Could you check a few things on this model? Use its own coordinates, in mm. A direction names the side the tool comes from. Coordinates: 2 decimals unless noted, no trailing zeros. Write each loop counter-clockwise with the first axis right and the second up, starting at its lowest first coordinate (ties: lowest second). Pieces come first, ordered by that corner, then holes.
```python
from build123d import *
from OCP.BRepFilletAPI import BRepFilletAPI_MakeChamfer

# Parameters (mm, degrees)
BOSS_EXTRUDE1_DEPTH     = 55
CUT_EXTRUDE2_DEPTH      = 206.91260281973967
CUT_EXTRUDE2_DEPTH_BACK = 206.91260281973967
SKETCH2_W               = 100.40000000000003
SKETCH2_H               = 20.399999999999995
CUT_EXTRUDE3_DEPTH      = 19
CUT_EXTRUDE4_DEPTH      = 206.91260281973967
CUT_EXTRUDE4_DEPTH_BACK = 206.91260281973967
CUT_EXTRUDE12_DEPTH     = 206.91260281973967
BOSS_EXTRUDE2_DEPTH     = 55
CHAMFER1_SIZE           = 14.54
CHAMFER1_SIZE2          = 14.538004892432124
CHAMFER8_SIZE           = 14.54
CHAMFER8_SIZE2          = 14.541995746543376
CHAMFER10_SIZE          = 3
CHAMFER10_SIZE2         = 1.732050807568882
BOSS_EXTRUDE4_DEPTH     = 55
SKETCH39_R              = 1.949999999999999
CUT_EXTRUDE13_DEPTH     = 11
SKETCH40_R              = 2.3000000000000105
SKETCH40_R_2            = 2.2999999999999985
CUT_EXTRUDE14_DEPTH     = 212.78054679313647
SKETCH41_R              = 2.2999999999999927
SKETCH41_R_2            = 2.300000000000006
CUT_EXTRUDE15_DEPTH     = 212.78054679313647
SKETCH42_R              = 5.000000000000005
SKETCH42_R_2            = 5.000000000000004
SKETCH42_R_3            = 4.99999999999999
CUT_EXTRUDE16_DEPTH     = 214.57902518739957
CHAMFER6_SIZE           = 1
CHAMFER13_SIZE          = 2
CHAMFER14_SIZE          = 4
SKETCH35_R              = 2.3
SKETCH35_R_2            = 2.3000000000000007
CUT_EXTRUDE11_DEPTH     = 157.6455394949968
CHAMFER15_SIZE          = 1
CHAMFER12_SIZE          = 2


with BuildPart() as part:
    # Sketch1 → Boss-Extrude1 (new body)
    with BuildSketch(Plane(origin=(0, 0, 0), x_dir=(1, 0, 0), z_dir=(0, 1, 0))):
        Polygon((0, 0), (149.99999999999937, 0), (74.99999999999966, 129.903810567666), align=None)
    extrude(amount=-BOSS_EXTRUDE1_DEPTH)

    # Sketch4 → Cut-Extrude2 (cut, two sides: drawn at the far end of the back side and taken through both)
    with BuildSketch(Plane(origin=(0, 0, 0), x_dir=(1, 0, 0), z_dir=(0, 1, 0)).offset(-CUT_EXTRUDE2_DEPTH_BACK)):
        Polygon((58.51197371389166, 45.56656990669255), (40.84586371751368, 35.365170120590925), (51.0472635036153, 17.699060124212945), (68.71337349999328, 27.90045991031457), align=None)
    extrude(amount=CUT_EXTRUDE2_DEPTH + CUT_EXTRUDE2_DEPTH_BACK, mode=Mode.SUBTRACT)

    # Sketch2 → Cut-Extrude3 (cut)
    with BuildSketch(Plane(origin=(0, 0, 0), x_dir=(1, 0, 0), z_dir=(0, 1, 0))):
        Polygon((109.19704525612455, 138.33483042000623), (58.99704525612457, 51.385879880048556), (41.33012701892186, 61.58587988004866), (91.53012701892203, 148.5348304200062), align=None)
        with Locations((124.20000000000002, 15.199999999999998)):
            Rectangle(SKETCH2_W, SKETCH2_H)
    extrude(amount=-CUT_EXTRUDE3_DEPTH, mode=Mode.SUBTRACT)

    # Sketch27 → Cut-Extrude4 (cut, two sides: drawn at the far end of the back side and taken through both)
    with BuildSketch(Plane(origin=(0, 0, 0), x_dir=(1, 0, 0), z_dir=(0, 1, 0)).offset(-CUT_EXTRUDE4_DEPTH_BACK)):
        Polygon((263.2126301054118, 395.09764853640723), (92.55144818336423, 99.50381056766552), (63.425446507958185, 49.05609584452599), (74.19851948196656, 30.4), (132.44855181663485, 30.400000000000006), (473.7709156607301, 30.40000000000005), (1064.9585915982134, 371.72236384409547), (854.4003060428951, 736.4200123805026), align=None)
    extrude(amount=CUT_EXTRUDE4_DEPTH + CUT_EXTRUDE4_DEPTH_BACK, mode=Mode.SUBTRACT)

    # Sketch36 → Cut-Extrude12 (cut, through all)
    with BuildSketch(Plane(origin=(0, 0, 0), x_dir=(1, 0, 0), z_dir=(0, 1, 0))):
        Polygon((0, 0), (27.744423358828314, 48.054750884192224), (55.49392370110368, 0), align=None)
    extrude(amount=-CUT_EXTRUDE12_DEPTH, mode=Mode.SUBTRACT)

    # Sketch37 → Boss-Extrude2 (add)
    with BuildSketch(Plane(origin=(0, 0, 0), x_dir=(1, 0, 0), z_dir=(0, 1, 0))):
        Polygon((34.51566032896974, 36.328770172306804), (61.707613950845634, 52.03092474503183), (75.90956267267339, 27.436928475564457), (48.717609050797485, 11.734773902839414), align=None)
        Polygon((58.51197371389166, 45.56656990669254), (40.84586371751368, 35.365170120590925), (51.0472635036153, 17.699060124212945), (68.71337349999328, 27.90045991031457), align=None, mode=Mode.SUBTRACT)
    extrude(amount=BOSS_EXTRUDE2_DEPTH)

    # Chamfer1
    chamfer1_edges = [part.edges().sort_by_distance(p)[0] for p in [
        (27.744423358828314, -27.499999999999996, -48.054750884192224),
    ]]
    chamfer1_side = [part.faces().sort_by_distance(p)[0] for p in [
        (41.61831404888806, -8.880686552520038, -24.028863834628613),
    ]]
    chamfer(chamfer1_edges, length=CHAMFER1_SIZE, length2=CHAMFER1_SIZE2, reference=chamfer1_side[0])

    # Chamfer8
    chamfer8_edges = [part.edges().sort_by_distance(p)[0] for p in [
        (55.49392370110368, -27.5, 0),
    ]]
    chamfer8_side = [part.faces().sort_by_distance(p)[0] for p in [
        (43.89644444718681, -5.451869149628209, -20.083748159692625),
    ]]
    chamfer(chamfer8_edges, length=CHAMFER8_SIZE, length2=CHAMFER8_SIZE2, reference=chamfer8_side[0])

    # Chamfer10: one chamfer whose edges measure the first distance from different faces: ONE call of the kernel's chamfer builder (chamfer() names one face for all edges)
    chamfer10_edges_1 = [part.edges().sort_by_distance(p)[0] for p in [
        (41.619173529966076, 55, -24.027375442095966),
    ]]
    chamfer10_side_1 = [part.faces().sort_by_distance(p)[0] for p in [
        (41.61917352996608, 4.8e-16, -24.02737544209596),
    ]]
    chamfer10_edges_2 = [part.edges().sort_by_distance(p)[0] for p in [
        (68.80858831175951, 55, -39.73392661029814),
    ]]
    chamfer10_side_2 = [part.faces().sort_by_distance(p)[0] for p in [
        (68.81005262159329, 3.7755355816469027, -39.731390815296024),
    ]]
    chamfer10 = BRepFilletAPI_MakeChamfer(part.part.solid().wrapped)
    for e in chamfer10_edges_1:
        chamfer10.Add(CHAMFER10_SIZE, CHAMFER10_SIZE2, e.wrapped, chamfer10_side_1[0].wrapped)  # the first distance lies on this face
    for e in chamfer10_edges_2:
        chamfer10.Add(CHAMFER10_SIZE, CHAMFER10_SIZE2, e.wrapped, chamfer10_side_2[0].wrapped)  # the first distance lies on this face
    add(Compound.cast(chamfer10.Shape()), mode=Mode.REPLACE)

    # Sketch28 → Boss-Extrude4 (add)
    with BuildSketch(Plane(origin=(0, 0, 0), x_dir=(1, 0, 0), z_dir=(0, 1, 0))):
        Polygon((63.4254465079582, 49.05609584452599), (78.17205931308985, 74.59797846255982), (85.54536553049708, 61.82937401563315), align=None)
        Polygon((103.69444359160526, 30.4), (74.19851948196656, 30.4), (96.31843850450542, 43.173278171107164), align=None)
    extrude(amount=-BOSS_EXTRUDE4_DEPTH)

    # Sketch39 → Cut-Extrude13 (cut)
    with BuildSketch(Plane(origin=(90.92850733429839, 0, -52.5072047814054), x_dir=(-0.5000686169657652, 0, -0.8659857841361757), z_dir=(0.8659857841361756, 0, -0.5000686169657651))):
        with Locations((-21.499999999999993, -4.999999999999996)):
            Circle(SKETCH39_R)
        with Locations((21.500000000000004, -4.999999999999996)):
            Circle(SKETCH39_R)
        with Locations((21.50000000000001, -47.99999999999999)):
            Circle(SKETCH39_R)
        with Locations((-21.499999999999986, -47.99999999999999)):
            Circle(SKETCH39_R)
    extrude(amount=-CUT_EXTRUDE13_DEPTH, mode=Mode.SUBTRACT)

    # Sketch40 → Cut-Extrude14 (cut, through all)
    with BuildSketch(Plane(origin=(0, -19, 0), x_dir=(1, 0, 0), z_dir=(0, 1, 0))):
        with Locations(Location((76.27572409168204, 101.7134295108992, 0), (0, 0, 270))):
            Circle(SKETCH40_R)
        with Locations(Location((57.66358613752323, 69.47626093681517, 0), (0, 0, 270))):
            Circle(SKETCH40_R_2)
    extrude(amount=-CUT_EXTRUDE14_DEPTH, mode=Mode.SUBTRACT)

    # Sketch41 → Cut-Extrude15 (cut, through all)
    with BuildSketch(Plane(origin=(0, -19, 0), x_dir=(1, 0, 0), z_dir=(0, 1, 0))):
        with Locations(Location((89, 15.2, 0), (0, 0, 270))):
            Circle(SKETCH41_R)
        with Locations(Location((126.22427590831714, 15.199999999999998, 0), (0, 0, 270))):
            Circle(SKETCH41_R_2)
    extrude(amount=-CUT_EXTRUDE15_DEPTH, mode=Mode.SUBTRACT)

    # Sketch42 → Cut-Extrude16 (cut, through all)
    with BuildSketch(Plane(origin=(0, -24, 0), x_dir=(1, 0, 0), z_dir=(0, 1, 0))):
        with Locations(Location((76.27572409168204, 101.7134295108992, 0), (0, 0, 270))):
            Circle(SKETCH42_R)
        with Locations(Location((57.66358613752323, 69.47626093681517, 0), (0, 0, 270))):
            Circle(SKETCH42_R)
        with Locations(Location((89, 15.2, 0), (0, 0, 270))):
            Circle(SKETCH42_R_2)
        with Locations(Location((126.22427590831714, 15.199999999999998, 0), (0, 0, 270))):
            Circle(SKETCH42_R_3)
    extrude(amount=-CUT_EXTRUDE16_DEPTH, mode=Mode.SUBTRACT)

    # Chamfer6
    chamfer6_edges = [part.edges().sort_by_distance(p)[0] for p in [
        (63.612673606942465, -55.00000000000001, -36.73351490850356),
        (59.88031850180429, -55.00000000000001, -22.79976001726376),
        (45.94656361056448, -55.00000000000001, -26.532115122401926),
        (49.67891871570267, -55.00000000000001, -40.465870013641734),
    ]]
    chamfer(chamfer6_edges, length=CHAMFER6_SIZE)

    # Chamfer13
    chamfer13_edges = [part.edges().sort_by_distance(p)[0] for p in [
        (76.27572409168204, -55, -106.7134295108992),
        (57.66358613752323, -55, -74.47626093681517),
        (89, -55, -20.200000000000003),
        (126.22427590831714, -55, -20.19999999999999),
    ]]
    chamfer(chamfer13_edges, length=CHAMFER13_SIZE)

    # Chamfer14
    chamfer14_edges = [part.edges().sort_by_distance(p)[0] for p in [
        (63.425446507958185, -27.5, -49.05609584452599),
        (74.19851948196656, -27.5, -30.4),
    ]]
    chamfer(chamfer14_edges, length=CHAMFER14_SIZE)

    # Sketch35 → Cut-Extrude11 (cut, through all)
    with BuildSketch(Plane(origin=(45.94656361056447, 0, -26.53211512240196), x_dir=(-0.5000686169657652, 0, -0.8659857841361754), z_dir=(0.8659857841361756, 0, -0.5000686169657653))):
        with Locations((3.67e-15, -30)):
            Circle(SKETCH35_R)
        Circle(SKETCH35_R_2)
        with Locations((-3.67e-15, 30)):
            Circle(SKETCH35_R)
    extrude(amount=CUT_EXTRUDE11_DEPTH, mode=Mode.SUBTRACT)

    # Chamfer15
    chamfer15_edges = [part.edges().sort_by_distance(p)[0] for p in [
        (102.65511640214558, -4.999999999999996, -32.19983814341209),
        (81.15216587261767, -47.99999999999999, -69.43722686126765),
        (102.65511640214558, -47.99999999999999, -32.199838143412094),
        (81.15216587261767, -4.999999999999996, -69.43722686126763),
    ]]
    chamfer(chamfer15_edges, length=CHAMFER15_SIZE)

    # Chamfer12
    chamfer12_edges = [part.edges().sort_by_distance(p)[0] for p in [
        (141.2242759083171, -55, -15.200000000000003),
        (35.01442342727759, -55, -48.054175012116296),
        (41.61917352996607, -55.00000000000001, -24.027375442095966),
        (110.01795972382322, -55, 0),
        (59.12942272903427, -55.00000000000001, -6.295716650669986),
        (81.85871242179346, -55, -68.21367623909649),
        (118.07149770412005, -55, -30.400000000000002),
        (86.99045056150834, -55, -37.786776319485114),
        (100.00644104805534, -55, -36.78663908555358),
        (76.21737758749998, -55, -56.44287216401109),
        (68.81198299496236, -55, -39.728047922263),
        (66.15755531016205, -55, -48.324261510185174),
        (74.93035381630737, -55, -33.13210880220387),
        (55.006712902522075, -55, -95.27442150452332),
        (83.77572409168201, -55, -114.70381056766587),
        (85.36175374822707, -55.00000000000001, -87.05089451511276),
    ]]
    chamfer(chamfer12_edges, length=CHAMFER12_SIZE)


solid = part.part
```
Item 1: If I drill on line 1 along X through (y, z) = (-20.85, -15.2); line 2 along Z through (x, y) = (92, -7); line 3 along Z through (x, y) = (83, -22), over which ranges is the centre line in solid material (lowest first)?
Item 2: I want a section at B-B, the plane x = 113.5. List the corners of the cut face in (y, z) for me, then the cut area to 3 significant figures.
Item 3: Which directions (+Z, -Z, +X, -X, +Y, -Y) give clear straight access to the entire face, cutting with the end or side of a thin tool? Please do faces 1 (the flat face through (63.961, -54.493, -37.116)), 2 (the flat face through (92.17, -47.97, -28.36)), 3 (the flat face through (48.175, 27.115, -44.216)), 4 (the flat face through (74, -9, -15)), 5 (the flat face through (118, -27, -30.4)).
Item 4: I want a section at D-D, the plane z = -58. List the corners of the cut face in (x, y) for me, then the cut area to 3 significant figures.
Item 5: Will these pins go through, and if not, where does the flat tip stop? pin 1 Ø7.5 at (x, z) = (57.66, -69.48) entering from +Y; pin 2 Ø6 at (x, z) = (93.5, -106.5) entering from +Y; pin 3 Ø5 at (x, y) = (133.5, -24.5) entering from -Z; pin 4 Ø8 at (x, z) = (125, -14.5) entering from -Y.
Item 6: I want a section at A-A, the plane y = -11.5. List the corners of the cut face in (x, z) for me.
Item 7: If we mould it in two halves opening along Y, with no side actions, what happens to faces 6 (the flat face through (41.71, -1.23, -23.87)), 7 (the flat face through (92.17, -4.97, -28.36)), 8 (the flat face through (57, -24, -67))? For each: released by +Y, released by -Y, zero draft, split by the parting line, or undercut.
Item 8: I want a section at C-C, the plane y = 47.5. List the corners of the cut face in (x, z) for me.
Taken from the geometry:
1. line 1: x = 46.72 to 86.7, 91.3 to 123.92, 128.52 to 141.22
1. line 2: z = -100.46 to -98.55, -40.68 to -25.4, -5 to 0
1. line 3: z = -116.05 to -82.96, -66.24 to -60.36, -35.48 to 0
2. outline: (-55, -28.4) - (-53, -30.4) - (0, -30.4) - (0, -25.4) - (-19, -25.4) - (-19, -5) - (0, -5) - (0, 0) - (-53, 0) - (-55, -2) - close
2. area: 1,280 mm2
3. face 1: -Y
3. face 2: none
3. face 3: -Z, -X, +Y
3. face 4: +X, +Y
3. face 5: -Z, +X, +Y, -Y
4. outline: (35.01, -53) - (37.01, -55) - (74.91, -55) - (78.91, -53) - (78.91, 0) - (62.82, 0) - (62.82, -19) - (47.54, -19) - (47.54, 0) - (35.01, 0) - close
4. area: 2,120 mm2
5. pin 1: stops at y = -19
5. pin 2: passes through
5. pin 3: stops at z = -30.4
5. pin 4: stops at y = -53.41
6. outline: (35.01, -60.65) - (75, -129.9) - (77.89, -124.9) - (41.33, -61.59) - (59, -51.39) - (89.66, -104.5) - (92.55, -99.5) - (78.17, -74.6) - (85.55, -61.83) - (66.89, -51.06) - (65.43, -45.59) - (72.2, -33.86) - (77.66, -32.4) - (96.32, -43.17) - (103.69, -30.4) - (132.45, -30.4) - (135.34, -25.4) - (74, -25.4) - (74, -5) - (147.11, -5) - (150, 0) - (70.04, 0) - (48.22, -12.59) - (35.02, -35.46) - close; hole (40.85, -35.37) - (58.51, -45.57) - (68.71, -27.9) - (51.05, -17.7) - close
7. face 6: zero draft
7. face 7: undercut
7. face 8: released by -Y
8. outline: (35.02, -36.62) - (61.71, -52.03) - (75.91, -27.44) - (49.21, -12.02) - (48.22, -12.59) - (35.02, -35.46) - close; hole (40.85, -35.37) - (58.51, -45.57) - (68.71, -27.9) - (51.05, -17.7) - close
